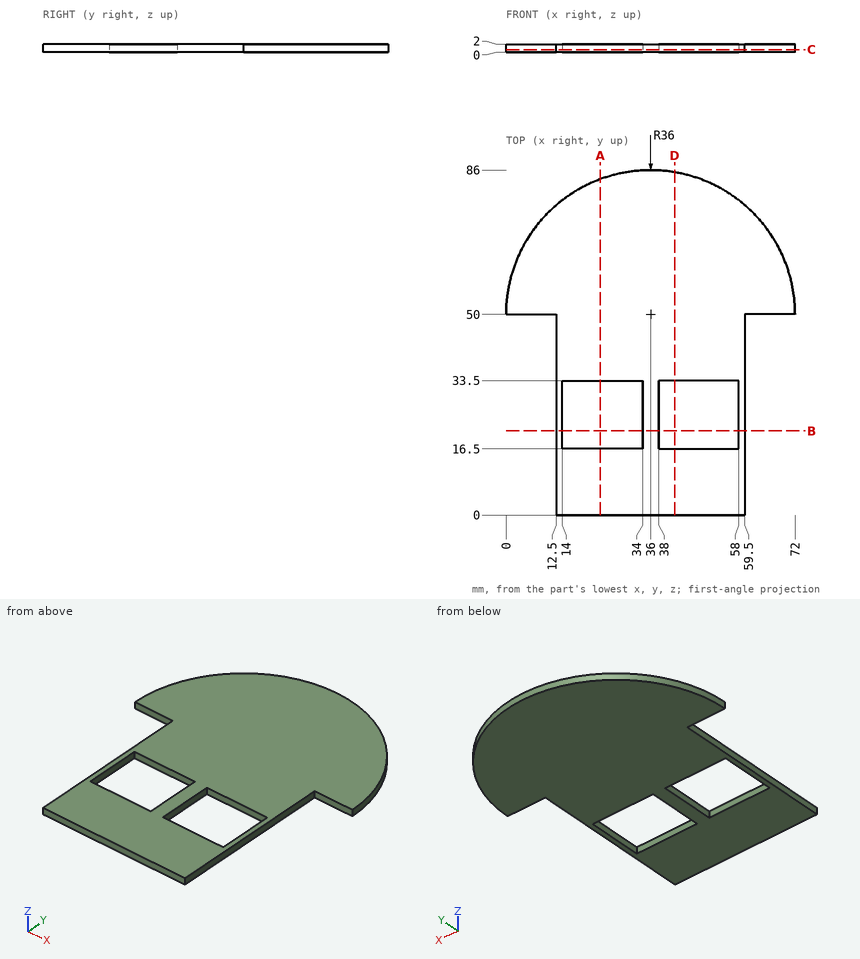
Study the drawing (mm; zero at the part's minimum x, y, z) and answer. Round coordinates to 2 decimals unless told otherwise and drop trailing zeros. Write each loop counter-clockwise with the first axis right and the second up, starting at its lowest first coordinate (ties: lowest second). Pieces come first, ordered by that corner, then holes. Notation, with made-up numbers: (50, 41.25) -> (89, 41.25) arc R32 ccw to (89, 73.25) -> close; hole circle Ø5 at (48.25, 56.5). An arc over 180 degrees is marked (long way). Write each question's results on one line, items separated by ' | '.
Item 1: A cutting plane is placed at A-A, the plane x = 23.5. Determine the outline of the cut face in (y, z), plus the area to 3 significant figures.
Result set:
outline: (0, 0) -> (16.5, 0) -> (16.5, 2) -> (0, 2) -> close; (33.5, 0) -> (83.76, 0) -> (83.76, 2) -> (33.5, 2) -> close | area: 134 mm^2
Item 2: A cutting plane is placed at C-C, the plane z = 0.6. Determine the outline of the cut face in (x, y).
Result set:
outline: (0, 50) -> (12.5, 50) -> (12.5, 0) -> (59.5, 0) -> (59.5, 50) -> (72, 50) arc R36 ccw to start; hole (14, 16.5) -> (34, 16.5) -> (34, 33.5) -> (14, 33.5) -> close; hole (38, 16.5) -> (58, 16.5) -> (58, 33.5) -> (38, 33.5) -> close
Item 3: Find the intervals of material crossed by line 1 along X through (y, z) = (7, 1); line 2 along Y through (x, z) = (16, 1.55); line 3 along Y through (x, z) = (32, 0.5), in increasing order. Write a range as [from, to].
Result set:
line 1: [12.5, 59.5] | line 2: [0, 16.5], [33.5, 79.93] | line 3: [0, 16.5], [33.5, 85.78]
Item 4: Flat-ended cylindrical pins translate along their axes: P1, Ø1, axis at x = 51.5, z = 1, coming from the +Y side; P2, Ø8, axis at x = 46, y = 28.5, coming from the -Z side; P3, Ø0.6, axis at y = 22.5, z = 1, coming from the +X side; P4, Ø0.6, axis at y = 21, z = 1, coming from the -X side. Find the tip coordinate at first contact, or state that the pin passes through.
Result set:
P1: y = 82.73 | P2: through | P3: x = 59.5 | P4: x = 12.5
Item 5: A cutting plane is placed at D-D, the plane x = 42. Determine the outline of the cut face in (y, z).
Result set:
outline: (0, 0) -> (16.5, 0) -> (16.5, 2) -> (0, 2) -> close; (33.5, 0) -> (85.5, 0) -> (85.5, 2) -> (33.5, 2) -> close
Item 6: A cutting plane is placed at B-B, the plane y = 21. Determine the outline of the cut face in (x, z).
Result set:
outline: (12.5, 0) -> (14, 0) -> (14, 2) -> (12.5, 2) -> close; (34, 0) -> (38, 0) -> (38, 2) -> (34, 2) -> close; (58, 0) -> (59.5, 0) -> (59.5, 2) -> (58, 2) -> close
